from build123d import *

# Parameters (mm, degrees)
F1_DEPTH = 6.35
F2_W     = 3.175
F2_H     = 6.35
F2_H_2   = 6.349999
F2_H_3   = 6.350001
F3_DEPTH = 2.54


with BuildPart() as f1:
    # F0 (on Top) → F1 (new body)
    with BuildSketch(Plane.XY):
        with BuildLine():
            Line((0, 36.501117), (0, 31.421117))
            ThreePointArc((0, 31.421117), (1.188232, 26.402755), (1.5875, 21.261117))
            Line((1.5875, 21.261117), (1.5875, -56.137312))
            ThreePointArc((1.5875, -56.137312), (3.175, -59.518786), (4.7625, -56.137312))
            Line((4.7625, -56.137312), (4.7625, 21.261117))
            ThreePointArc((4.7625, 21.261117), (7.983405, 30.631791), (0, 36.501117))
        make_face()
        with BuildLine():
            ThreePointArc((-1.5875, 21.261117), (-1.188232, 26.402755), (0, 31.421117))
            Line((0, 31.421117), (0, 36.501117))
            ThreePointArc((0, 36.501117), (-7.983405, 30.631791), (-4.7625, 21.261117))
            Line((-4.7625, 21.261117), (-4.7625, -56.137312))
            ThreePointArc((-4.7625, -56.137312), (-3.175, -59.518786), (-1.5875, -56.137312))
            Line((-1.5875, -56.137312), (-1.5875, 21.261117))
        make_face()
    extrude(amount=F1_DEPTH)

    # F2 (on face) → F3 (join)
    with BuildSketch(Plane.XY.offset(6.35)):
        with Locations((-3.175, 18.086117)):
            Rectangle(F2_W, F2_H)
        with Locations((3.175, 11.736117)):
            Rectangle(F2_W, F2_H)
        with Locations((-3.175, 5.386117)):
            Rectangle(F2_W, F2_H)
        with Locations((3.175, -0.963883)):
            Rectangle(F2_W, F2_H)
        with Locations((-3.175, -7.313883)):
            Rectangle(F2_W, F2_H)
        with Locations((3.175, -13.663883)):
            Rectangle(F2_W, F2_H)
        with Locations((-3.175, -20.013883)):
            Rectangle(F2_W, F2_H)
        with Locations((3.175, -26.363883)):
            Rectangle(F2_W, F2_H)
        with Locations((-3.175, -32.713883)):
            Rectangle(F2_W, F2_H)
        with Locations((3.175, -39.063883)):
            Rectangle(F2_W, F2_H)
        with Locations((-3.175, -45.413882)):
            Rectangle(F2_W, F2_H_2)
        with Locations((3.175, -51.763882)):
            Rectangle(F2_W, F2_H_3)
        with BuildLine():
            Line((-1.5875, -56.137312), (-1.5875, -54.938883))
            Line((-1.5875, -54.938883), (-4.7625, -54.938883))
            Line((-4.7625, -54.938883), (-4.7625, -56.137312))
            ThreePointArc((-4.7625, -56.137312), (-3.175, -59.518786), (-1.5875, -56.137312))
        make_face()
    extrude(amount=F3_DEPTH)


solid = f1.part
Can you work these out from the model? Positions are in its coordinate system, mm. A direction names the side the tool comes from. Coordinates: 2 decimals unless noted, no trailing zeros. Order: outer loops, then holes, each group sorted by start corner. A loop starts at its lowest first (then second) coordinate and runs counter-clockwise, first axis right, second up. Notation, with made-up numbers: (87, -20.5) - (140, -20.5) arc R23 ccw to (140, -6.5) - close; hole circle Ø4 at (3.5, 0.5). An arc over 180 degrees is marked (long way). Answer as a JSON object with one key per item and string values. Group by question number.
Q1. Will these pins go through, and if not, where does the flat tip stop? P1, Ø2.5, axis at x = -3, y = 10.5, coming from the +Z side; P2, Ø1.3, axis at x = 3.5, z = 8, coming from the -Y side; P3, Ø0.8, axis at x = 2.5, z = 7, coming from the +Y side.
Q2. Imagine slicing it at C-C (x = 3). Please give me the cut outline in (y, z).
Q3. We'd pull the mould along Y, two halves only. Please class faces 1 (the face through (2, 28, 6.35)), 2 (the face through (3, -48.589, 8)): +Y half, -Y half, draft (parallel to the pull), parting line (faces both ways), or undercut.
Q4. Imagine slicing it at A-A (y = -11.5). Please give me the cut outline in (x, z).
Q5. I need wall thicknesses on line 1 (X direction, y = -34, z = 0.75); line 2 (X direction, y = 20.5, z = 7.25); line 3 (Z direction, x = 3, y = -4.5). Which ranges of each line are inside material? Lowest first, please. Write a range as from..to.
Q6. On a 3-axis mill with a long thin cutter (end or side, diameter ignored), from which of +Z, -Z, +X, -X, +Y, -Y can I reach the whole of each face in a straight line? I mean faces 3 (the face through (-3, -54.939, 8)), 4 (the face through (-3, -33, 8.89)), 5 (the face through (3, -4.139, 8)). Say none if no direction works.
Q7. Imagine slicing it at B-B (z = 4.5). Please give me the cut outline in (x, y) (1 decimal).
Determined:
{
 "1": {"P1": "stops at z = 6.35", "P2": "stops at y = -54.94", "P3": "stops at y = 14.91"},
 "2": {"outline": "(-59.51, 0) - (35.94, 0) - (35.94, 6.35) - (14.91, 6.35) - (14.91, 8.89) - (8.56, 8.89) - (8.56, 6.35) - (2.21, 6.35) - (2.21, 8.89) - (-4.14, 8.89) - (-4.14, 6.35) - (-10.49, 6.35) - (-10.49, 8.89) - (-16.84, 8.89) - (-16.84, 6.35) - (-23.19, 6.35) - (-23.19, 8.89) - (-29.54, 8.89) - (-29.54, 6.35) - (-35.89, 6.35) - (-35.89, 8.89) - (-42.24, 8.89) - (-42.24, 6.35) - (-48.59, 6.35) - (-48.59, 8.89) - (-54.94, 8.89) - (-54.94, 6.35) - (-59.51, 6.35) - close"},
 "3": {"face 1": "draft", "face 2": "undercut"},
 "4": {"outline": "(-4.76, 0) - (-1.59, 0) - (-1.59, 6.35) - (-4.76, 6.35) - close; (1.59, 0) - (4.76, 0) - (4.76, 8.89) - (1.59, 8.89) - close"},
 "5": {"line 1": "x = -4.76..-1.59, 1.59..4.76", "line 2": "x = -4.76..-1.59", "line 3": "z = 0..6.35"},
 "6": {"face 3": "+Z, -X", "face 4": "+Z, +X, -X, +Y, -Y", "face 5": "+Z, +X"},
 "7": {"outline": "(-4.8, -56.1) arc R2.1 ccw (long way) to (-1.6, -56.1) - (-1.6, 21.3) arc R33.3 cw to (0, 31.4) arc R33.3 cw to (1.6, 21.3) - (1.6, -56.1) arc R2.1 ccw (long way) to (4.8, -56.1) - (4.8, 21.3) arc R8.4 ccw to (0, 36.5) arc R8.4 ccw to (-4.8, 21.3) - close"}
}
